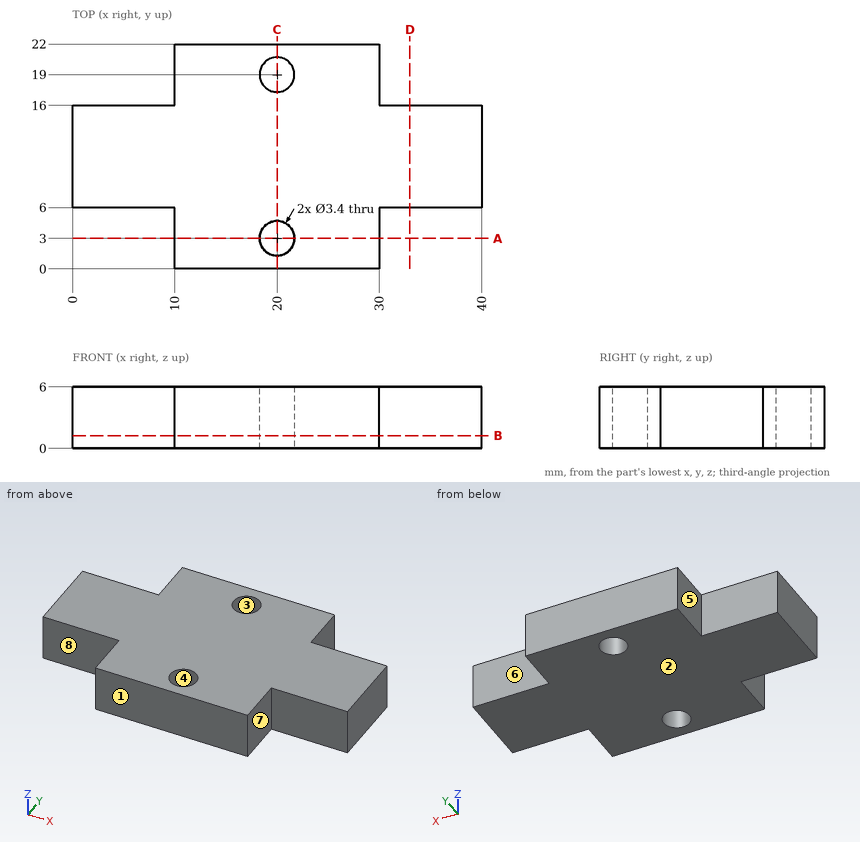
Verification items for this drawing (mm, ordinates from the low corner). A direction names the side the tool comes from. Round coordinates to 2 decimals unless told otherwise and drop trailing zeros. Loops run counter-clockwise (first coordinate to the right, second up) from the corner with the lowest first, then second, coordinate; pieces in that order, holes last. Notation, with made-up numbers: (46.25, 38.25) -> (91.25, 38.25) arc R20 cw to (91.25, 55.25) -> close; hole circle Ø3 at (60.25, 86). An arc over 180 degrees is marked (long way). Answer in a Markdown table with one row per item.
Q1. Sectioned sample at A-A on y = 3. Enter the section's corners in (x, z).
Data:
| item | result |
|---|---|
| outline | (10, 0) -> (18.3, 0) -> (18.3, 6) -> (10, 6) -> close; (21.7, 0) -> (30, 0) -> (30, 6) -> (21.7, 6) -> close |
Q2. Sectioned sample at B-B on z = 1.25. Enter the section's corners in (x, y).
Data:
| item | result |
|---|---|
| outline | (0, 6) -> (10, 6) -> (10, 0) -> (30, 0) -> (30, 6) -> (40, 6) -> (40, 16) -> (30, 16) -> (30, 22) -> (10, 22) -> (10, 16) -> (0, 16) -> close; hole circle Ø3.4 at (20, 3); hole circle Ø3.4 at (20, 19) |
Q3. Set-up check for the marked faces 5, 6, 7 and 8: record each of +Z, -Z, +X, -X, +Y, -Y from which the full face is reachable in a straight line by a thin tool's end or side.
Data:
| item | result |
|---|---|
| face 5 | +Z, -Z, -X, +Y |
| face 6 | +Z, -Z, +X, +Y |
| face 7 | +Z, -Z, +X, -Y |
| face 8 | +Z, -Z, -X, -Y |
Q4. Go/stop test with flat-tipped pins: P1, Ø3, axis at y = 18, z = 3.5, coming from the +X side; P2, Ø3, axis at x = 36.5, z = 4, coming from the -Y side; P3, Ø1.5, axis at y = 4.5, z = 4, coming from the -X side. Record where each tip stops, or that it passes through.
Data:
| item | result |
|---|---|
| P1 | stops at x = 30 |
| P2 | stops at y = 6 |
| P3 | stops at x = 10 |
Q5. Sectioned sample at D-D on x = 33. Enter the section's corners in (y, z), then the cut area to 3 significant figures.
Data:
| item | result |
|---|---|
| outline | (6, 0) -> (16, 0) -> (16, 6) -> (6, 6) -> close |
| area | 60.0 mm^2 |
Q6. Release check for a two-part mould opening along Y. For the marked faces 1, 2, 3 and 4 record: released by +Y, released by -Y, zero draft, split by the parting line, or undercut.
Data:
| item | result |
|---|---|
| face 1 | released by -Y |
| face 2 | zero draft |
| face 3 | undercut |
| face 4 | undercut |
Q7. Thickness scan on L1, parallel to Y at x = 20, z = 4.65; L2, parallel to X at y = 3, z = 1.75; L3, parallel to Y at x = 3.5, z = 1.4. Record the ranges inside material, lowest first.
Data:
| item | result |
|---|---|
| L1 | y = 0 to 1.3, 4.7 to 17.3, 20.7 to 22 |
| L2 | x = 10 to 18.3, 21.7 to 30 |
| L3 | y = 6 to 16 |
Q8. Sectioned sample at C-C on x = 20. Enter the section's corners in (y, z).
Data:
| item | result |
|---|---|
| outline | (0, 0) -> (1.3, 0) -> (1.3, 6) -> (0, 6) -> close; (4.7, 0) -> (17.3, 0) -> (17.3, 6) -> (4.7, 6) -> close; (20.7, 0) -> (22, 0) -> (22, 6) -> (20.7, 6) -> close |
